```python
from build123d import *

# Parameters (mm, degrees)
F0_W     = 279.4
F0_H     = 279.4
F1_DEPTH = 12.7
F2_R     = 6.874077
F2_W     = 21.59
F2_H     = 21.59
F3_DEPTH = 3.96875
F4_W     = 256.317572
F4_H     = 256.317572
F4_W_2   = 224.567598
F4_H_2   = 224.567598
F5_DEPTH = 7.9375


with BuildPart() as f1:
    # F0 (on Top) → F1 (new body)
    with BuildSketch(Plane.XY):
        Rectangle(F0_W, F0_H)
    extrude(amount=-F1_DEPTH)

    # F2 (on Top) → F3 (cut)
    with BuildSketch(Plane.XY):
        with Locations((-56.914803, -94.826)):
            Circle(F2_R)
        with Locations((-56.914803, -69.426)):
            Circle(F2_R)
        with Locations((-56.914803, -44.026)):
            Circle(F2_R)
        with Locations((-56.914803, -18.626)):
            Circle(F2_R)
        with Locations((-56.914803, 6.774)):
            Circle(F2_R)
        with Locations((-56.914803, 32.174)):
            Circle(F2_R)
        with Locations((-56.914803, 57.574)):
            Circle(F2_R)
        with Locations((-31.514803, -94.826)):
            Circle(F2_R)
        with Locations((-31.514803, -69.426)):
            Circle(F2_R)
        with Locations((-31.514803, -44.026)):
            Circle(F2_R)
        with Locations((-31.514803, -18.626)):
            Circle(F2_R)
        with Locations((-31.514803, 6.774)):
            Circle(F2_R)
        with Locations((-31.514803, 32.174)):
            Circle(F2_R)
        with Locations((-31.514803, 57.574)):
            Circle(F2_R)
        with Locations((-6.114803, -94.826)):
            Circle(F2_R)
        with Locations((-6.114803, -69.426)):
            Circle(F2_R)
        with Locations((-6.114803, -44.026)):
            Circle(F2_R)
        with Locations((-6.114803, -18.626)):
            Circle(F2_R)
        with Locations((-6.114803, 6.774)):
            Circle(F2_R)
        with Locations((-6.114803, 32.174)):
            Circle(F2_R)
        with Locations((-6.114803, 57.574)):
            Circle(F2_R)
        with Locations((19.285197, -94.826)):
            Circle(F2_R)
        with Locations((19.285197, -69.426)):
            Circle(F2_R)
        with Locations((19.285197, -44.026)):
            Circle(F2_R)
        with Locations((19.285197, -18.626)):
            Circle(F2_R)
        with Locations((19.285197, 6.774)):
            Circle(F2_R)
        with Locations((19.285197, 32.174)):
            Circle(F2_R)
        with Locations((19.285197, 57.574)):
            Circle(F2_R)
        with Locations((44.685197, -94.826)):
            Circle(F2_R)
        with Locations((44.685197, -69.426)):
            Circle(F2_R)
        with Locations((44.685197, -44.026)):
            Circle(F2_R)
        with Locations((44.685197, -18.626)):
            Circle(F2_R)
        with Locations((44.685197, 6.774)):
            Circle(F2_R)
        with Locations((44.685197, 32.174)):
            Circle(F2_R)
        with Locations((44.685197, 57.574)):
            Circle(F2_R)
        with Locations((70.085197, -94.826)):
            Circle(F2_R)
        with Locations((70.085197, -69.426)):
            Circle(F2_R)
        with Locations((70.085197, -44.026)):
            Circle(F2_R)
        with Locations((70.085197, -18.626)):
            Circle(F2_R)
        with Locations((70.085197, 6.774)):
            Circle(F2_R)
        with Locations((70.085197, 32.174)):
            Circle(F2_R)
        with Locations((70.085197, 57.574)):
            Circle(F2_R)
        with Locations((95.485197, -94.826)):
            Circle(F2_R)
        with Locations((95.485197, -69.426)):
            Circle(F2_R)
        with Locations((95.485197, -44.026)):
            Circle(F2_R)
        with Locations((95.485197, -18.626)):
            Circle(F2_R)
        with Locations((95.485197, 6.774)):
            Circle(F2_R)
        with Locations((95.485197, 32.174)):
            Circle(F2_R)
        with Locations((95.485197, 57.574)):
            Circle(F2_R)
        with Locations((-95.014803, -94.826)):
            Circle(F2_R)
        with Locations((95.485197, 95.674)):
            Circle(F2_R)
        with Locations((70.085197, 95.674)):
            Circle(F2_R)
        with Locations((44.685197, 95.674)):
            Circle(F2_R)
        with Locations((19.285197, 95.674)):
            Circle(F2_R)
        with Locations((-6.114803, 95.674)):
            Circle(F2_R)
        with Locations((-31.514803, 95.674)):
            Circle(F2_R)
        with Locations((-56.914803, 95.674)):
            Circle(F2_R)
        with Locations((-95.014803, -69.426)):
            Circle(F2_R)
        with Locations((-95.014803, -44.026)):
            Circle(F2_R)
        with Locations((-95.014803, -18.626)):
            Circle(F2_R)
        with Locations((-95.014803, 6.774)):
            Circle(F2_R)
        with Locations((-95.014803, 32.174)):
            Circle(F2_R)
        with Locations((-95.014803, 57.574)):
            Circle(F2_R)
        with Locations((-95.014803, 95.674)):
            Rectangle(F2_W, F2_H)
    extrude(amount=-F3_DEPTH, mode=Mode.SUBTRACT)

    # F4 (on Top) → F5 (cut)
    with BuildSketch(Plane.XY):
        Rectangle(F4_W, F4_H)
        Rectangle(F4_W_2, F4_H_2, mode=Mode.SUBTRACT)
    extrude(amount=-F5_DEPTH, mode=Mode.SUBTRACT)


solid = f1.part
```
Check sheet for the modelled part. Datum: model origin and axes. Units: mm. A direction names the side the tool comes from. Give positions to 0.01 mm unless a question says otherwise; leave off trailing zeros. Write each loop counter-clockwise with the first axis right and the second up, starting at its lowest first coordinate (ties: lowest second). Pieces come first, ordered by that corner, then holes.
Item 1: Cross-section at A-A (x = 122). Enter the section's corners in (y, z).
Item 2: Draft check along X on faces 1 (the face through (19, 96, -3.969)), 2 (the face through (-95, -19, -3.969)), 3 (the face through (-11, -134, 0)). Enter one of: released by +X, released by -X, zero draft, split by the parting line, or undercut.
Item 3: Gauge pin test, flat end, axial feed: pin 1 (4 mm diameter, centred on x = -9, y = -43, fed in from +Z). Record the tip position at first contact, or that the pin passes through.
Item 4: Access from +Z, -Z, +X, -X, +Y, -Y to the whole of each face (thin tool, end or side, straight path). Record for faces 4 (the face through (-2, -139.7, -6)), 5 (the face through (70, -19, -3.969)).
Item 5: Scan lines: L1, parallel to Y at x = 5.5, z = -2.25; L2, parallel to X at y = -127.5, z = -6.25. Record each from-to range of solid material in increasing order.
Item 6: Cross-section at B-B (y = 81). Enter the section's corners in (x, z), and give its area (3 significant figures).
Report:
1. outline: (-139.7, -12.7) - (139.7, -12.7) - (139.7, 0) - (128.16, 0) - (128.16, -7.94) - (-128.16, -7.94) - (-128.16, 0) - (-139.7, 0) - close
2. face 1: undercut
2. face 2: undercut
2. face 3: zero draft
3. pin 1: stops at z = -3.97
4. face 4: +Z, -Z, +X, -X, -Y
4. face 5: +Z
5. L1: y = -139.7 to -128.16, -112.28 to 112.28, 128.16 to 139.7
5. L2: x = -139.7 to -128.16, 128.16 to 139.7
6. outline: (-139.7, -12.7) - (139.7, -12.7) - (139.7, 0) - (128.16, 0) - (128.16, -7.94) - (112.28, -7.94) - (112.28, 0) - (-112.28, 0) - (-112.28, -7.94) - (-128.16, -7.94) - (-128.16, 0) - (-139.7, 0) - close
6. area: 3,300 mm2
